Could you check a few things on this drawing? It's one solid part, dimensions in mm from its lowest x, y, z. A direction names the side the tool comes from. Give positions to 0.01 mm unless a question says otherwise; leave off trailing zeros. Loops run counter-clockwise (first coordinate to the right, second up) from the corner with the lowest first, then second, coordinate; pieces in that order, holes last. Notation, with made-up numbers: (-39, 38) - (-30, 38) arc R5 ccw to (-30, 43) - close; hole circle Ø3 at (84, -35). An arc over 180 degrees is marked (long way). Answer as a JSON object with one key per item and string values.
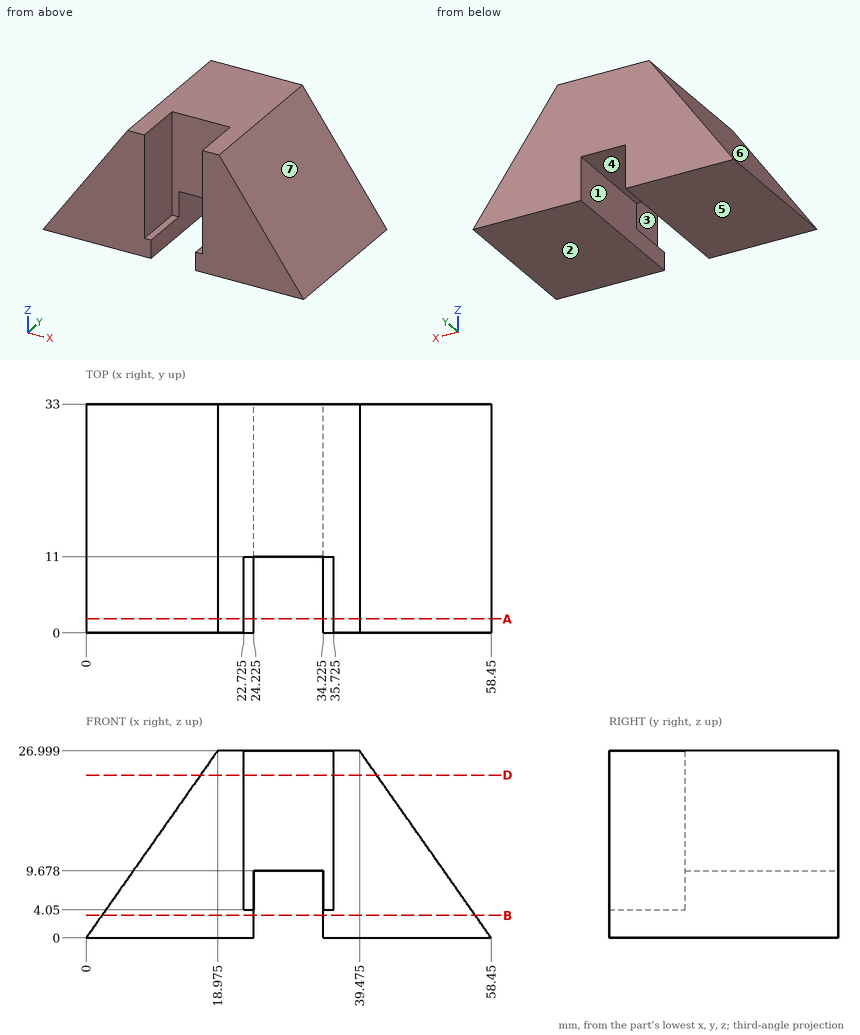
1) I need wall thicknesses on L1, parallel to Y at x = 34, z = 17.5; L2, parallel to X at y = 13, z = 6 (1 decimal); L3, parallel to X at y = 28, z = 7 (1 decimal). Which ranges of each line are inside material? Lowest first, please.
Check sheet entries:
{"L1": "11 to 33", "L2": "4.2 to 24.2, 34.2 to 54.2", "L3": "4.9 to 24.2, 34.2 to 53.5"}
2) Imagine slicing it at B-B on z = 3.25. Write out the boundary of the cut face in (x, y) (1 decimal).
Check sheet entries:
{"outline": "(2.3, 0) - (24.2, 0) - (24.2, 33) - (2.3, 33) - close; (34.2, 0) - (56.2, 0) - (56.2, 33) - (34.2, 33) - close"}
3) Imagine slicing it at A-A on y = 2. Write out the boundary of the cut face in (x, z) (3 decimals).
Check sheet entries:
{"outline": "(0, 0) - (24.225, 0) - (24.225, 4.05) - (22.725, 4.05) - (22.725, 26.999) - (18.975, 26.999) - close; (34.225, 0) - (58.45, 0) - (39.475, 26.999) - (35.725, 26.999) - (35.725, 4.05) - (34.225, 4.05) - close"}
4) If we mould it in two halves opening along X, with no side actions, what happens to the marked faces 4, 5, 6 and 7? For each: released by +X, released by -X, zero draft, split by the parting line, or undercut.
Check sheet entries:
{"face 4": "undercut", "face 5": "zero draft", "face 6": "released by -X", "face 7": "released by +X"}
5) Which directions (+Z, -Z, +X, -X, +Y, -Y) give clear straight access to the entire face, cutting with the end or side of a thin tool? Please do the marked faces 1, 2 and 3.
Check sheet entries:
{"face 1": "-Z, +Y, -Y", "face 2": "-Z, +X, -X, +Y, -Y", "face 3": "+Z, -Y"}
6) I'm going to push flat-ended pins straight in: P1, Ø2, axis at y = 27.5, z = 18, coming from the -X side; P2, Ø4, axis at x = 7, y = 10.5, coming from the -Z side; P3, Ø5.5, axis at y = 5.5, z = 20.5, coming from the -X side (1 decimal); P4, Ø7.5, axis at y = 23, z = 5.5, coming from the +X side. Where does each tip first touch, or does it pass through?
Check sheet entries:
{"P1": "x = 11.95", "P2": "z = 0", "P3": "x = 12.5", "P4": "x = 57.22"}
7) Imagine slicing it at D-D on z = 23.5. Write out the boundary of the cut face in (x, y) (1 decimal), and give its area (3 significant figures).
Check sheet entries:
{"outline": "(16.5, 0) - (22.7, 0) - (22.7, 11) - (35.7, 11) - (35.7, 0) - (41.9, 0) - (41.9, 33) - (16.5, 33) - close", "area": "696 mm2"}
